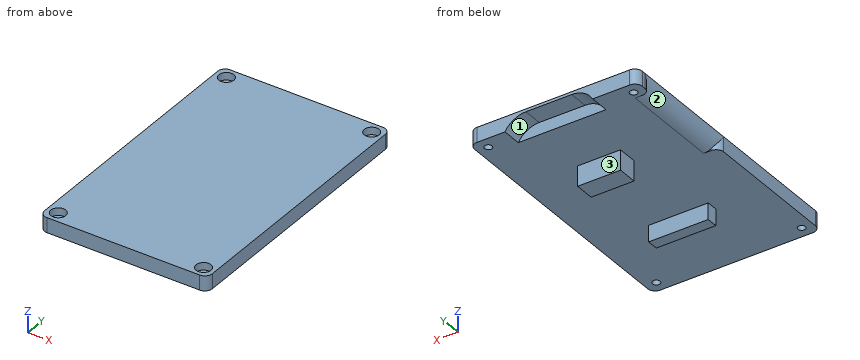
from build123d import *

# Parameters (mm, degrees)
SKETCH_1_W          = 22.5
SKETCH_1_H          = 36
EXTRUDE_1_DEPTH     = 2
SKETCH_9_R          = 1
CUT_EXTRUDE_3_DEPTH = 1
CUT_EXTRUDE_4_REACH = 145.222
SKETCH_10_R         = 0.5
FILLET_1_R          = 1
SKETCH_11_W         = 5.762947655
SKETCH_11_H         = 2.6557086
EXTRUDE_2_DEPTH     = 2.7
SKETCH_12_W         = 8
SKETCH_12_H         = 1.496173859
EXTRUDE_3_DEPTH     = 2.2
SKETCH_14_W         = 2
SKETCH_14_H         = 13.482091112
CUT_EXTRUDE_6_DEPTH = 0.0001
FILLET_3_R          = 2
CUT_EXTRUDE_7_DEPTH = 2.62
FILLET_7_R          = 1


with BuildPart() as part:
    # 草图1 → 凸台-拉伸1 (new body)
    with BuildSketch(Plane.XY):
        with Locations((-109.040086771, 59.72858385)):
            Rectangle(SKETCH_1_W, SKETCH_1_H)
    extrude(amount=EXTRUDE_1_DEPTH)

    # 草图9 → 切除-拉伸3 (cut)
    with BuildSketch(Plane.XY.offset(2)):
        with Locations((-99.290086771, 76.22858385)):
            Circle(SKETCH_9_R)
        with Locations((-99.290086771, 43.22858385)):
            Circle(SKETCH_9_R)
        with Locations((-118.790086771, 43.22858385)):
            Circle(SKETCH_9_R)
        with Locations((-118.790086771, 76.22858385)):
            Circle(SKETCH_9_R)
    extrude(amount=-CUT_EXTRUDE_3_DEPTH, mode=Mode.SUBTRACT)

    # 草图10 → 切除-拉伸4 (cut, up to next)
    with BuildSketch(Plane.XY.offset(1), mode=Mode.PRIVATE) as cut_extrude_4_sk1:
        with Locations((-118.790086771, 43.22858385)):
            Circle(SKETCH_10_R)
    cut_extrude_4_tool1 = extrude(cut_extrude_4_sk1.sketch, amount=-CUT_EXTRUDE_4_REACH, mode=Mode.PRIVATE) & part.part
    # 草图10 → 切除-拉伸4 (cut, up to next)
    with BuildSketch(Plane.XY.offset(1), mode=Mode.PRIVATE) as cut_extrude_4_sk2:
        with Locations((-99.290086771, 43.22858385)):
            Circle(SKETCH_10_R)
    cut_extrude_4_tool2 = extrude(cut_extrude_4_sk2.sketch, amount=-CUT_EXTRUDE_4_REACH, mode=Mode.PRIVATE) & part.part
    # 草图10 → 切除-拉伸4 (cut, up to next)
    with BuildSketch(Plane.XY.offset(1), mode=Mode.PRIVATE) as cut_extrude_4_sk3:
        with Locations((-99.290086771, 76.22858385)):
            Circle(SKETCH_10_R)
    cut_extrude_4_tool3 = extrude(cut_extrude_4_sk3.sketch, amount=-CUT_EXTRUDE_4_REACH, mode=Mode.PRIVATE) & part.part
    # 草图10 → 切除-拉伸4 (cut, up to next)
    with BuildSketch(Plane.XY.offset(1), mode=Mode.PRIVATE) as cut_extrude_4_sk4:
        with Locations((-118.790086771, 76.22858385)):
            Circle(SKETCH_10_R)
    cut_extrude_4_tool4 = extrude(cut_extrude_4_sk4.sketch, amount=-CUT_EXTRUDE_4_REACH, mode=Mode.PRIVATE) & part.part
    add(cut_extrude_4_tool1.solids().sort_by_distance((-118.790087, 43.228584, 1))[0], mode=Mode.SUBTRACT)
    add(cut_extrude_4_tool2.solids().sort_by_distance((-99.290087, 43.228584, 1))[0], mode=Mode.SUBTRACT)
    add(cut_extrude_4_tool3.solids().sort_by_distance((-99.290087, 76.228584, 1))[0], mode=Mode.SUBTRACT)
    add(cut_extrude_4_tool4.solids().sort_by_distance((-118.790087, 76.228584, 1))[0], mode=Mode.SUBTRACT)

    # 圆角1
    fillet_1_edges = [part.edges().sort_by_distance(p)[0] for p in [
        (-97.790086771, 41.72858385, 1),
        (-120.290086771, 41.72858385, 1),
        (-120.290086771, 77.72858385, 1),
        (-97.790086771, 77.72858385, 1),
    ]]
    fillet(fillet_1_edges, radius=FILLET_1_R)

    # 草图11 → 凸台-拉伸2 (add)
    with BuildSketch(Plane(origin=(0, 0, 0), x_dir=(-1, 0, 0), z_dir=(0, 0, -1))):
        with Locations((108.208612944, 66.20072955)):
            Rectangle(SKETCH_11_W, SKETCH_11_H)
    extrude(amount=EXTRUDE_2_DEPTH)

    # 草图12 → 凸台-拉伸3 (add)
    with BuildSketch(Plane(origin=(0, 0, 0), x_dir=(-1, 0, 0), z_dir=(0, 0, -1))):
        with Locations((109.081368677, 52.476670779)):
            Rectangle(SKETCH_12_W, SKETCH_12_H)
    extrude(amount=EXTRUDE_3_DEPTH)

    # 草图14 → 切除-拉伸6 (cut)
    with BuildSketch(Plane.ZY.offset(120.290086771)):
        with Locations((1, 68.480990424)):
            Rectangle(SKETCH_14_W, SKETCH_14_H)
    extrude(amount=-CUT_EXTRUDE_6_DEPTH, mode=Mode.SUBTRACT)

    # 圆角3
    # the kernel refuses this fillet: 2 mm, written as the material it takes off along each edge
    with BuildSketch(Plane(origin=(-120.289986771, 61.739944868, 0), x_dir=(1, 0, 0), z_dir=(0, 1, 0))) as fillet_3_piece_1:
        with BuildLine():
            CenterArc((FILLET_3_R, -FILLET_3_R), FILLET_3_R, 90, 90)
            Line((0, -FILLET_3_R), (0, 0))
            Line((0, 0), (FILLET_3_R, 0))
        make_face()
    extrude(amount=13.482091112, mode=Mode.SUBTRACT)

    # 草图16 → 切除-拉伸7 (cut)
    with BuildSketch(Plane(origin=(0, 77.72858385, 0), x_dir=(1, 0, 0), z_dir=(0, 1, 0))):
        with BuildLine():
            Line((-111.502300349, 4.875), (-105.366426438, 4.875))
            ThreePointArc((-105.366426438, 4.875), (-102.116426438, 1.625), (-105.366426438, -1.625))
            Line((-105.366426438, -1.625), (-111.502300349, -1.625))
            ThreePointArc((-111.502300349, -1.625), (-114.752300349, 1.625), (-111.502300349, 4.875))
        make_face()
    extrude(amount=-CUT_EXTRUDE_7_DEPTH, mode=Mode.SUBTRACT)

    # 圆角7
    # the kernel refuses this fillet: 1 mm, written as the material it takes off along each edge
    with BuildSketch(Plane(origin=(-120.290086771, 61.739944868, 4.5), x_dir=(0, -1, 0), z_dir=(0, 0, -1))) as fillet_7_piece_1_section:
        with BuildLine():
            CenterArc((FILLET_7_R, -FILLET_7_R), FILLET_7_R, 90, 90)
            Line((0, -FILLET_7_R), (0, 0))
            Line((0, 0), (FILLET_7_R, 0))
        make_face()
    fillet_7_piece_1 = extrude(amount=7, mode=Mode.PRIVATE)
    fillet_7_piece_1 = fillet_7_piece_1 - Plane(origin=(-118.289986771, 61.479548888, 2), x_dir=(1, 0, 0), z_dir=(0, -1, 0)) * Cylinder(2, 18, mode=Mode.PRIVATE)
    add(fillet_7_piece_1, mode=Mode.SUBTRACT)
    with BuildSketch(Plane(origin=(-120.290086771, 75.22203598, -2.5), x_dir=(1, 0, 0), z_dir=(0, 0, 1))) as fillet_7_piece_2_section:
        with BuildLine():
            CenterArc((FILLET_7_R, FILLET_7_R), FILLET_7_R, 180, 90)
            Line((0, FILLET_7_R), (0, 0))
            Line((0, 0), (FILLET_7_R, 0))
        make_face()
    fillet_7_piece_2 = extrude(amount=7, mode=Mode.PRIVATE)
    fillet_7_piece_2 = fillet_7_piece_2 - Plane(origin=(-118.289986771, 75.482431596, 2), x_dir=(1, 0, 0), z_dir=(0, -1, 0)) * Cylinder(2, 18, mode=Mode.PRIVATE)
    add(fillet_7_piece_2, mode=Mode.SUBTRACT)


solid = part.part
Can you work these out from the model? Positions are in its coordinate system, mm. Face numbers are marked on the shaded views. Give positions to 0.01 mm unless a question says otherwise; leave off trailing zeros. Order: outer loops, then holes, each group sorted by start corner. A loop starts at its lowest first (then second) coordinate and runs counter-clockwise, first axis right, second up. Notation, with made-up numbers: M -20.75,-3.75 L -10.75,-3.75 A17 ccw -10.75,22.25 Z; hole C 11,25.25 d9. An arc over 180 degrees is marked long. Use one line per item in the form item = value.
Item 1: If I drill on line 1 along Y through (x, z) = (-106.5, -0.5); line 2 along X through (y, z) = (67, -2.15); line 3 along Z through (x, y) = (-103.5, 60), over which ranges is the centre line in solid material (lowest first)? Write a range as [from, to].
Values follow:
line_1 = [51.73, 53.22], [64.87, 67.53]
line_2 = [-111.09, -105.33]
line_3 = [0, 2]
Item 2: If we section it at B-B, the plane y = 67: Write out the boundary of the cut face in (x, z), and give its area (3 significant figures).
Values follow:
outline = M -120.29,2 A2 ccw -118.29,0 L -111.09,0 L -111.09,-2.7 L -105.33,-2.7 L -105.33,0 L -97.79,0 L -97.79,2 Z
area = 59.7 mm^2
Item 3: If we section it at C-C, the plane x = -99.25: Write out the boundary of the cut face in (y, z).
Values follow:
outline = M 41.73,0 L 42.73,0 L 42.73,1 L 42.23,1 L 42.23,2 L 41.73,2 Z; M 43.73,0 L 75.73,0 L 75.73,1 L 75.23,1 L 75.23,2 L 44.23,2 L 44.23,1 L 43.73,1 Z; M 76.73,0 L 77.73,0 L 77.73,2 L 77.23,2 L 77.23,1 L 76.73,1 Z
Item 4: Thinking about a two-plate mould opening in Y: for the marked faces 1, 2 and 3, which applies, pulls with the +Y half, pulls with the -Y half, needs draft (parallel to the pull), parting line crosses it, or undercut?
Values follow:
face_1 = needs draft
face_2 = undercut
face_3 = pulls with the +Y half
Item 5: If we section it at D-D, the plane x = -109.5: Write out the boundary of the cut face in (y, z) (3 decimals).
Values follow:
outline = M 41.729,0 L 51.729,0 L 51.729,-2.2 L 53.225,-2.2 L 53.225,0 L 64.873,0 L 64.873,-2.7 L 67.529,-2.7 L 67.529,0 L 75.109,0 L 75.109,1.625 L 77.729,1.625 L 77.729,2 L 41.729,2 Z
Item 6: Will these pins go through, and if not, where does the flat tip stop? pin 1 Ø1.8 at (x, y) = (-118.79, 43.23) entering from -Z; pin 2 Ø1.8 at (x, z) = (-107.5, -1.5) entering from -Y; pin 3 Ø1.2 at (y, z) = (52.5, -1.5) entering from +X.
Values follow:
pin_1 = 0
pin_2 = 51.73
pin_3 = -105.08
Item 7: If we section it at A-A, the plane z = -0.9: Write out the boundary of the cut face in (x, y).
Values follow:
outline = M -113.08,51.73 L -105.08,51.73 L -105.08,53.22 L -113.08,53.22 Z; M -111.09,64.87 L -105.33,64.87 L -105.33,67.53 L -111.09,67.53 Z
